Geometry check sheet. Reference: the model listing, model coordinates, mm. Face numbers are marked on the shaded views. Round coordinates to 2 decimals unless told otherwise and drop trailing zeros. Write each loop counter-clockwise with the first axis right and the second up, starting at its lowest first coordinate (ties: lowest second). Pieces come first, ordered by that corner, then holes. Notation, with made-up numbers: (18, -12) -> (51, -12) arc R11 cw to (51, 4) -> close; hole circle Ø8 at (85, 52). An arc over 180 degrees is marked (long way). One line per question, with ' | ' between items.
```python
from build123d import *

# Parameters (mm, degrees)
F0_W          = 62
F0_H          = 20
F1_DEPTH      = 0.9
F3_DEPTH      = 50
F3_DEPTH_BACK = 20


with BuildPart() as f1:
    # F0 (on Top) → F1 (new body)
    with BuildSketch(Plane.XY):
        Rectangle(F0_W, F0_H)
    extrude(amount=F1_DEPTH)

    # F2 (on face) → F3 (join, two sides)
    with BuildSketch(Plane.XZ.offset(10)) as f3_sk:
        with BuildLine():
            ThreePointArc((-29.963264, 0.9), (-31.480364, 1.286107), (-32.372888, 0))
            Line((-32.372888, 0), (-31, 0))
            Line((-31, 0), (-31, 0.9))
            Line((-31, 0.9), (-29.963264, 0.9))
        make_face()
        with BuildLine():
            ThreePointArc((-29.627112, 0), (-29.713893, 0.480364), (-29.963264, 0.9))
            Line((-29.963264, 0.9), (-31, 0.9))
            Line((-31, 0.9), (-31, 0))
            Line((-31, 0), (-29.627112, 0))
        make_face()
        with BuildLine():
            ThreePointArc((32.372888, 0), (31.480364, 1.286107), (29.963264, 0.9))
            Line((29.963264, 0.9), (31, 0.9))
            Line((31, 0.9), (31, 0))
            Line((31, 0), (32.372888, 0))
        make_face()
        with BuildLine():
            Line((31, 0.9), (29.963264, 0.9))
            ThreePointArc((29.963264, 0.9), (29.713893, 0.480364), (29.627112, 0))
            Line((29.627112, 0), (31, 0))
            Line((31, 0), (31, 0.9))
        make_face()
    extrude(amount=F3_DEPTH)
    extrude(f3_sk.sketch, amount=-F3_DEPTH_BACK)


solid = f1.part
```
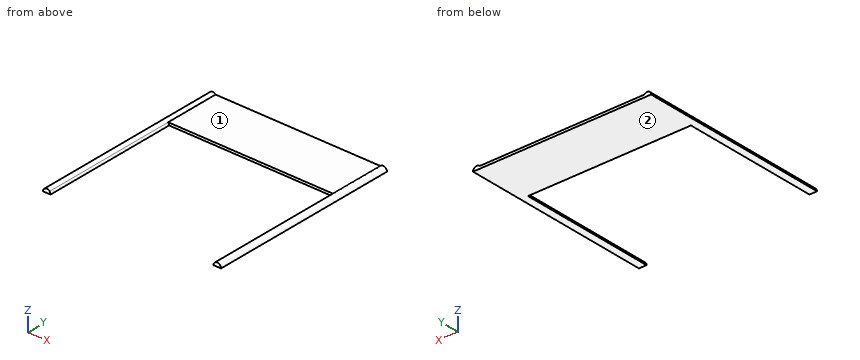
(1) Draft check along X on the marked faces 1 and 2. Enter one of: +X half, -X half, draft (parallel to the pull), parting line (faces both ways), or undercut.
Resolved:
face 1: undercut | face 2: draft
(2) Material ranges on line 1 (X direction, y = -17.5, z = 0.2); line 2 (Y direction, x = -20.5, z = 0.8); line 3 (Z direction, x = -18, y = -4.5), recorded low to high.
Resolved:
line 1: x = -32.36 to -29.64, 29.64 to 32.36 | line 2: y = -10 to 10 | line 3: z = 0 to 0.9
(3) Go/stop test with a flat-tipped pin: pin 1 (10 mm diameter, centred on x = 12.5, y = -9, fed in from +Z). Record where the tip stops, or that it passes through.
Resolved:
pin 1: stops at z = 0.9
(4) Sectioned sample at D-D on y = -5. Record the cut outline in (x, z).
Resolved:
outline: (-32.37, 0) -> (32.37, 0) arc R1.37 ccw to (29.96, 0.9) -> (-29.96, 0.9) arc R1.37 ccw to start
(5) Sectioned sample at B-B on z = 0.35. Record the cut outline in (x, y).
Resolved:
outline: (-32.33, -60) -> (-29.67, -60) -> (-29.67, -10) -> (29.67, -10) -> (29.67, -60) -> (32.33, -60) -> (32.33, 10) -> (-32.33, 10) -> close
(6) Sectioned sample at A-A on y = -47.5. Record the cut outline in (x, z).
Resolved:
outline: (-32.37, 0) -> (-29.63, 0) arc R1.37 ccw to (-29.96, 0.9) arc R1.37 ccw to start; (29.63, 0) -> (32.37, 0) arc R1.37 ccw to (29.96, 0.9) arc R1.37 ccw to start
(7) Sectioned sample at C-C on x = -16. Record the cut outline in (y, z), then the cut area to 3 significant figures.
Resolved:
outline: (-10, 0) -> (10, 0) -> (10, 0.9) -> (-10, 0.9) -> close | area: 18.0 mm2
